```python
from build123d import *

# Parameters (mm, degrees)
F0_R     = 15
F1_DEPTH = 2
F3_DEPTH = 1.05
F4_DEPTH = 0.05
F5_F1_R  = 0.4
F5_F2_R  = 0.4
F0_R_2   = 19.9891271991
F6_DEPTH = 50


with BuildPart() as f1:
    # F0 (on Top) → F1 (new body)
    with BuildSketch(Plane.XY):
        Circle(F0_R)
    extrude(amount=F1_DEPTH)

    # F2 (on Right) → F3 (join, symmetric)
    with BuildSketch(Plane.YZ):
        Polygon((-10, 12), (-15, 2), (15, 2), (10, 12), align=None)
    extrude(amount=F3_DEPTH, both=True)

    # F2 (on Right) → F4 (cut, symmetric)
    with BuildSketch(Plane.YZ):
        Polygon((-10, 12), (-15, 2), (15, 2), (10, 12), align=None)
    extrude(amount=F4_DEPTH, both=True, mode=Mode.SUBTRACT)

    # F5: fillet of radius 0.4 on 3 edges, made by hand

    # F5_f1
    f5_f1_edges = [f1.edges().sort_by_distance(p)[0] for p in [
        (-15, 0, 2),
    ]]
    fillet(f5_f1_edges, radius=F5_F1_R)

    # F5_f2
    f5_f2_edges = [f1.edges().sort_by_distance(p)[0] for p in [
        (10.9715541287, 10.2286362727, 2),
        (10.9715541287, -10.2286362727, 2),
    ]]
    fillet(f5_f2_edges, radius=F5_F2_R)

    # F0 (on Top) → F6 (cut)
    with BuildSketch(Plane.XY):
        Circle(F0_R_2)
        Circle(F0_R, mode=Mode.SUBTRACT)
    extrude(amount=F6_DEPTH, mode=Mode.SUBTRACT)


solid = f1.part
```
Geometry: final body of the model. Coordinates: model frame, mm. A direction names the side the tool comes from. Coordinates: 2 decimals unless noted, no trailing zeros. Order: outer loops, then holes, each group sorted by start corner. A loop starts at its lowest first (then second) coordinate and runs counter-clockwise, first axis right, second up. Notation, with made-up numbers: M 74,-32 L 94,-32 A29 ccw 94,-1 Z; hole C 51.5,87.25 d8. An arc over 180 degrees is marked long. Answer as CSV lines item,"result".
Q1. Section B-B on y = 0. Return the cut outline in (x, z), and give its area (3 significant figures).
Answers:
outline,"M -15,0 L 15,0 L 15,1.6 A0.4 ccw 14.6,2 L 1.05,2 L 1.05,12 L 0.05,12 L 0.05,2 L -0.05,2 L -0.05,12 L -1.05,12 L -1.05,2 L -14.6,2 A0.4 ccw -15,1.6 Z"
area,"79.9 mm^2"
Q2. Section C-C on z = 9.75. Return the cut outline in (x, y) (3 decimals), and give its area (3 significant figures).
Answers:
outline,"M -1.05,-11.125 L -0.05,-11.125 L -0.05,11.125 L -1.05,11.125 Z; M 0.05,-11.125 L 1.05,-11.125 L 1.05,11.125 L 0.05,11.125 Z"
area,"44.5 mm^2"
Q3. Section A-A on z = 7. Return the cut outline in (x, y).
Answers:
outline,"M -1.05,-12.5 L -0.05,-12.5 L -0.05,12.5 L -1.05,12.5 Z; M 0.05,-12.5 L 1.05,-12.5 L 1.05,12.5 L 0.05,12.5 Z"
Q4. First-contact query: P1, Ø1, axis at y = 10, z = 2, coming from the +X side; P2, Ø5, axis at y = 3, z = 5.5, coming from the -X side; P3, Ø8, axis at x = 6.5, y = -3.5, coming from the +Z side. Flat tips, straight axial feed; report the tip coordinate or a pass-through.
Answers:
P1,"stops at x = 11.52"
P2,"stops at x = -1.05"
P3,"stops at z = 2"
Q5. Line query: probe 1 along Z at (x, y) = (9, -4.75); probe 2 along Y at (x, z) = (-12.5, 1.25); probe 3 along Y at (x, z) = (1, 9). Output: solid intervals per line, ascending. Write a range as [from, to].
Answers:
probe 1,"z = [0, 2]"
probe 2,"y = [-8.29, 8.29]"
probe 3,"y = [-11.5, 11.5]"
Q6. Set-up query: faces 1 (the flat face through (6, 0, 2)), 2 (the flat face through (-6, 0, 2)), 3 (the cylindrical face through (-14.985, 0.66, 0.792)). Return all of +Z, -Z, +X, -X, +Y, -Y with unobstructed straight access to the full face (end or side cutting, diameter ignored); none if empty.
Answers:
face 1,"+Z, +X, +Y, -Y"
face 2,"+Z, -X, +Y, -Y"
face 3,"+Z, -Z"
